Could you check a few things on this model? Use its own coordinates, in mm. Face numbers are marked on the shaded views. A direction names the side the tool comes from. Coordinates: 2 decimals unless noted, no trailing zeros. Loops run counter-clockwise (first coordinate to the right, second up) from the corner with the lowest first, then second, coordinate; pieces in that order, holes last. Notation, with made-up numbers: M 50,45 L 109,45 A6 cw 109,56 Z; hole C -32.75,54.5 d10. An arc over 180 degrees is marked long. Write each question's results on one line, items separated by ' | '.
```python
from build123d import *

# Parameters (mm, degrees)
F0_W     = 40
F0_H     = 40
F0_R     = 2.25
F1_DEPTH = 5.5
F2_SIZE  = 2
F3_W     = 10
F3_H     = 15
F4_DEPTH = 20
F5_W     = 10
F5_H     = 10
F6_DEPTH = 25
F7_SIZE  = 1.5


with BuildPart() as f1:
    # F0 (on Front) → F1 (new body)
    with BuildSketch(Plane.XZ):
        with Locations((20, 20)):
            Rectangle(F0_W, F0_H)
        with Locations((9.999904, 9.999904)):
            Circle(F0_R, mode=Mode.SUBTRACT)
        with Locations((30.000096, 9.999904)):
            Circle(F0_R, mode=Mode.SUBTRACT)
        with Locations((9.999904, 30.000096)):
            Circle(F0_R, mode=Mode.SUBTRACT)
        with Locations((30.000096, 30.000096)):
            Circle(F0_R, mode=Mode.SUBTRACT)
    extrude(amount=F1_DEPTH)

    # F2
    f2_edges = [f1.edges().sort_by_distance(p)[0] for p in [
        (7.749904, -5.5, 30.000096),
        (27.750096, -5.5, 30.000096),
        (27.750096, -5.5, 9.999904),
        (7.749904, -5.5, 9.999904),
    ]]
    chamfer(f2_edges, length=F2_SIZE)

    # F3 (on face) → F4 (join)
    with BuildSketch(Plane.XZ.offset(5.5)):
        with Locations((20, 7.5)):
            Rectangle(F3_W, F3_H)
    extrude(amount=F4_DEPTH)

    # F5 (on face) → F6 (join)
    with BuildSketch(Plane.XY.offset(15)):
        with Locations((20, -20.5)):
            Rectangle(F5_W, F5_H)
    extrude(amount=F6_DEPTH)

    # F7
    f7_edges = [f1.edges().sort_by_distance(p)[0] for p in [
        (20, -25.5, 40),
        (25, -20.5, 40),
        (20, -15.5, 40),
        (15, -20.5, 40),
    ]]
    chamfer(f7_edges, length=F7_SIZE)


solid = f1.part
```
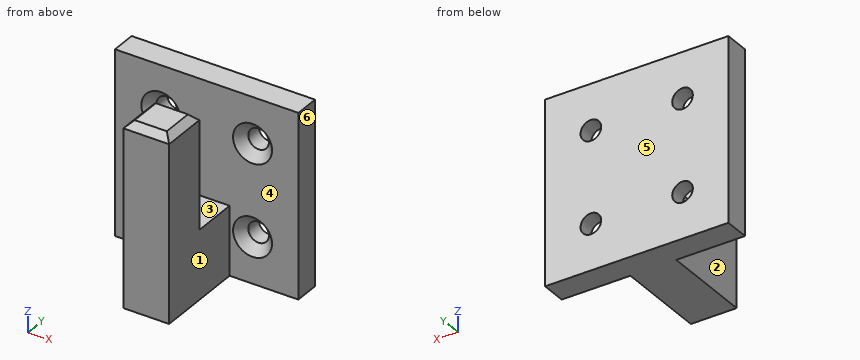
(1) Imagine slicing it at B-B, the plane y = -17.75. List the corners of the cut face in (x, z) for me.
Reported:
outline: M 15,0 L 25,0 L 25,38.5 L 23.5,40 L 16.5,40 L 15,38.5 Z
(2) Imagine slicing it at A-A, the plane z = 35. List the corners of the cut face in (x, y) for me.
Reported:
outline: M 0,-5.5 L 40,-5.5 L 40,0 L 0,0 Z; M 15,-25.5 L 25,-25.5 L 25,-15.5 L 15,-15.5 Z
(3) Which directions (+Z, -Z, +X, -X, +Y, -Y) give clear straight access to the entire face, cutting with the end or side of a thin tool? Please do the marked faces 1, 2 and 3.
Reported:
face 1: +Z, -Z, +X, -Y | face 2: +Z, -Z, -X, -Y | face 3: +Z, +X, -X
(4) Imagine slicing it at D-D, the plane y = -2. List the corners of the cut face in (x, z) for me, and give its area (3 significant figures).
Reported:
outline: M 0,0 L 40,0 L 40,40 L 0,40 Z; hole C 10,10 d4.5; hole C 10,30 d4.5; hole C 30,10 d4.5; hole C 30,30 d4.5 | area: 1,540 mm2
(5) Will these pins go through, and if not, where does the flat tip stop? P1, Ø8, axis at x = 22, y = -8.5, coming from the +Z side; P2, Ø3, axis at y = -18.5, z = 27, coming from the -X side; P3, Ø7, axis at x = 30, z = 10, coming from the -Y side; P4, Ø1.5, axis at x = 29.5, z = 25.5, coming from the -Y side.
Reported:
P1: stops at z = 40 | P2: stops at x = 15 | P3: stops at y = -4.75 | P4: stops at y = -5.5
(6) Please list where these lines run through material, in increasing order: probe 1 along Y at (x, z) = (22.5, 29); probe 2 along Z at (x, y) = (9.5, -5); probe 3 along Y at (x, z) = (7, 24.5). Write a range as from..to.
Reported:
probe 1: y = -25.5..-15.5, -5.5..0 | probe 2: z = 0..6.28, 13.72..26.28, 33.72..40 | probe 3: y = -5.5..0
(7) If we mould it in two halves opening along Y, with no side actions, what happens to the marked faces 4, 5 and 6? For each: released by +Y, released by -Y, zero draft, split by the parting line, or undercut.
Reported:
face 4: undercut | face 5: released by +Y | face 6: zero draft
(8) Imagine slicing it at C-C, the plane x = 18.5. List the corners of the cut face in (y, z) for me, and give its area (3 significant figures).
Reported:
outline: M -25.5,0 L 0,0 L 0,40 L -5.5,40 L -5.5,15 L -15.5,15 L -15.5,38.5 L -17,40 L -24,40 L -25.5,38.5 Z | area: 768 mm2
